Work out the finished part from the listing and answer in its coordinate system (mm). Face numbers are marked on the shaded views. A direction names the side the tool comes from. Give positions to 0.01 mm unless a question says otherwise; leave off trailing zeros. Write each loop counter-clockwise with the first axis right and the second up, starting at its lowest first coordinate (ties: lowest second). Pieces come first, ordered by that corner, then holes. Notation, with made-up numbers: (57, 82) - (74, 82) arc R30 ccw to (74, 109) - close; hole circle Ø11 at (80, 6). An arc over 180 degrees is marked (long way). Write item = value, one per line.
Autodesk Inventor part; units mm, degrees
ref_plane "YZ Plane" through (0, 0, 0) normal (1, 0, 0) x (0, 1, 0)
ref_plane "XZ Plane" through (0, 0, 0) normal (0, 1, 0) x (-1, 0, 0)
ref_plane "XY Plane" through (0, 0, 0) normal (0, 0, 1) x (1, 0, 0)
sketch "Sketch1" plane through (0, 0, 0) normal (0, 1, 0) x (-1, 0, 0)
  line L0 (-20, 7.5) -> (20, 7.5)
  line L1 (20, 7.5) -> (20, -7.5)
  line L2 (20, -7.5) -> (-20, -7.5)
  line L3 (-20, -7.5) -> (-20, 7.5)
  line L4 (-20, 7.5) -> (20, -7.5) construction
  line L5 (20, 7.5) -> (-20, -7.5) construction
  line L6 (20, 7.5) -> (40, 7.5)
  line L7 (40, 7.5) -> (40, -7.5)
  line L8 (40, -7.5) -> (20, -7.5)
  line L9 (20, -7.5) -> (20, 7.5)
  line L10 (20, 10) -> (40, 10)
  line L11 (40, 10) -> (40, -10)
  line L12 (40, -10) -> (20, -10)
  line L13 (20, -10) -> (20, 10)
  line L14 (20, 10) -> (40, -10) construction
  line L15 (40, 10) -> (20, -10) construction
  point P0 (0, 0)
  point P1 (30, 0)
  point P2 (20, -7.5)
  point P3 (40, -7.5)
  point P4 (20, 7.5)
  dimension "d0" = 40
  dimension "d1" = 15
  dimension "d2" = 20
  dimension "d3" = 20
  dimension "d4" = 20
extrude "Extrusion1" add sketch "Sketch1" along normal mid plane 10 contours L0 L1 L2 L3 | L6 L7 L8 L1
extrude "Extrusion2" add sketch "Sketch1" along normal mid plane 20 contours L6 L7 L8 L1 | L13 L10 L11 L6 | L8 L11 L12 L13
sketch "Sketch3" plane through (-40, -10, 10) normal (-1, 0, 0) x (0, 0, 1)
  circle A0 centre (-10, 10) radius 5
  dimension "d12" = 10
sketch "Sketch4" plane through (-40, 10, 10) normal (0, 0, 1) x (1, 0, 0)
  line L0 (20, 0) -> (20, -20)
  line L1 (0, 0) -> (20, 0)
  line L2 (0, -20) -> (0, 0)
  line L3 (20, -20) -> (0, -20)
  circle A0 centre (10, -10) radius 5
  point P0 (40, -10)
  dimension "d13" = 10
sketch "Sketch2" plane through (0, 10, 0) normal (0, 1, 0) x (1, 0, 0)
  line L0 (-20, -10) -> (-20, 10)
  line L1 (-20, 10) -> (-40, 10)
  line L2 (-40, 10) -> (-40, -10)
  line L3 (-40, -10) -> (-20, -10)
  circle A0 centre (-30, 0) radius 5
  point P0 (0, 0)
  dimension "d9" = 10
extrude "Extrusion3" cut sketch "Sketch2" against normal blind 5 contours A0
extrude "Extrusion4" cut sketch "Sketch3" against normal blind 5
extrude "Extrusion5" cut sketch "Sketch4" against normal blind 5 contours A0
sketch "Sketch5" plane through (0, -5, 0) normal (0, -1, 0) x (1, 0, 0)
  line L0 (-20, 7.5) -> (-20, -7.5)
  line L1 (-20, -7.5) -> (20, -7.5)
  line L2 (20, -7.5) -> (20, 7.5)
  line L3 (20, 7.5) -> (-20, 7.5)
  line L4 (20, 0) -> (-20, 0)
  circle A0 centre (5, 0) radius 1.5
  point P0 (0, 0)
  dimension "d18" = 3
  dimension "d19" = 15
extrude "Extrusion6" cut sketch "Sketch5" against normal blind 5 contours A0 L4 | L4 A0
properties part number "calibration_tool"
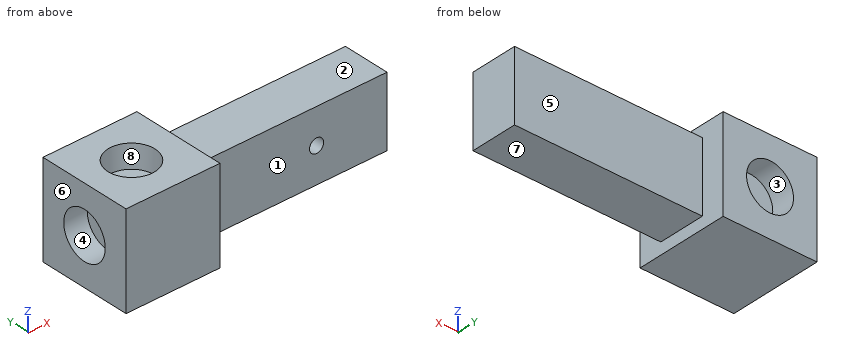
1. Find section C-C, the plane x = 5. Give the vertices of the cut face in (y, z).
Solution:
outline = (-5, -7.5) - (5, -7.5) - (5, 7.5) - (-5, 7.5) - (-5, 1.5) - (0, 1.5) - (0, -1.5) - (-5, -1.5) - close
2. Find section A-A, the plane y = 8. Give the vertices of the cut face in (x, z), then the cut area to 3 significant figures.
Solution:
outline = (-40, -10) - (-20, -10) - (-20, 10) - (-40, 10) - close; hole circle Ø10 at (-30, 0)
area = 321 mm^2
3. Straight lines are drawn through the part: line 1 (Z direction, x = 5, y = -1.7); line 2 (X direction, y = 0, z = 8.35); line 3 (Y direction, x = -38.45, z = 0). For each, find the intervals that lie inside material, in ascending order.
Solution:
line_1 = -7.5 to -1.5, 1.5 to 7.5
line_2 = -40 to -35, -25 to -20
line_3 = -10 to -5, 5 to 10
4. Find section D-D, the plane y = 2.5. Give the vertices of the cut face in (x, z).
Solution:
outline = (-40, -10) - (-20, -10) - (-20, -7.5) - (20, -7.5) - (20, 7.5) - (-20, 7.5) - (-20, 10) - (-25.67, 10) - (-25.67, 5) - (-34.33, 5) - (-34.33, 10) - (-40, 10) - (-40, 4.33) - (-35, 4.33) - (-35, -4.33) - (-40, -4.33) - close
5. Find section B-B, the plane z = 4. Give the vertices of the cut face in (x, y).
Solution:
outline = (-40, -10) - (-20, -10) - (-20, -5) - (20, -5) - (20, 5) - (-20, 5) - (-20, 10) - (-27, 10) - (-27, 5) - (-33, 5) - (-33, 10) - (-40, 10) - (-40, 3) - (-35, 3) - (-35, -3) - (-40, -3) - close
6. Given pin 1 (0.9 mm diameter, centred on x = 5.5, z = -0.5, fed in from -Y); pin 2 (10 mm diameter, centred on x = 1, z = 3.5, fed in from -Y); pin 3 (8 mm diameter, centred on x = 2.5, y = 0.5, fed in from +Z); pin 4 (11.5 mm diameter, centred on y = 0, z = 0, fed in from -X), each flat-ended and moving along its own axis, determine where each tip first touches the part or whether it passes through.
Solution:
pin_1 = 0
pin_2 = -5
pin_3 = 7.5
pin_4 = -40
7. A tool of negligible diameter and unlimited length cuts with its end or side. For the marked faces 1, 2, 3, 4 and 5, from which of +Z, -Z, +X, -X, +Y, -Y can it reach the whole face along a straight path? Write none if from no direction.
Solution:
face_1 = +Z, -Z, +X, -Y
face_2 = +Z, +X, +Y, -Y
face_3 = +Y
face_4 = -X
face_5 = +Z, -Z, +X, +Y
8. For a pull along X with two mould halves and no side action, classify the marked faces 6, 7 and 8 as pulls with the +X half, pulls with the -X half, needs draft (parallel to the pull), parting line crosses it, or undercut.
Solution:
face_6 = pulls with the -X half
face_7 = needs draft
face_8 = undercut
